Read the model definition and answer for the solid it produces. Units are mm, in the model's axes. Coordinates: 2 decimals unless noted, no trailing zeros. Write each loop counter-clockwise with the first axis right and the second up, starting at its lowest first coordinate (ties: lowest second). Pieces come first, ordered by that corner, then holes.
(1) The part is cut by section B-B, the plane z = 29.5. State how many separate pieces and enclosed holes the cut face has, and give its area (3 significant figures).
(2) The part is cut by section C-C, the plane x = 0. Determine the outline of the cut face in (y, z).
(3) Straight lines are drawn through the part: line 1 along Y through (x, z) = (34, 27.75); line 2 along Y through (x, z) = (-16, 29.25); line 3 along X through (y, z) = (-34, 20). For each, find the intervals that lie inside material, in ascending order.
(4) Given pin 1 (7 mm diameter, centred on x = 34, y = 16, fed in from -Z); pin 2 (2.5 mm diameter, centred on x = 34, y = 16, fed in from +Z); pin 3 (1.5 mm diameter, centred on x = -41.5, z = 22, fed in from +Y); pin 4 (5 mm diameter, centred on y = -11.5, z = 22, fed in from +X), each flat-ended and moving along its own axis, determine where each tip first touches the part or whether it passes through.
(5) The part is cut by section A-A, the plane y = 0. Determine the outline of the cut face in (x, z), and give its area (3 significant figures).
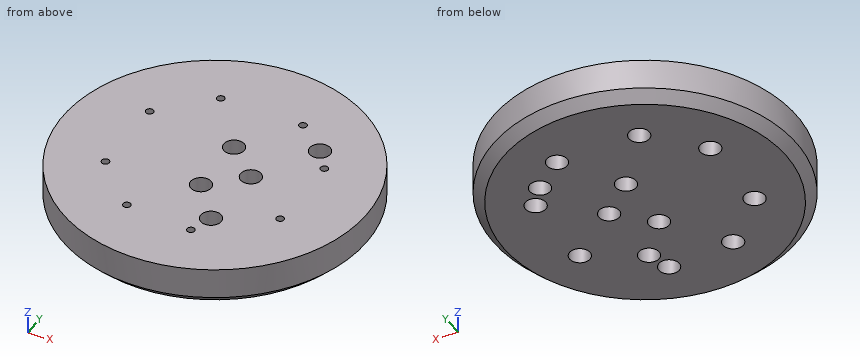
```python
from build123d import *

# Parameters (mm, degrees)
CYLINDER1648_R     = 4
CYLINDER1648_DEPTH = 100
CYLINDER1647_R     = 4
CYLINDER1647_DEPTH = 100
CYLINDER1631_R     = 1.5
CYLINDER1631_DEPTH = 100
CYLINDER1632_R     = 1.5
CYLINDER1632_DEPTH = 100
CYLINDER1633_R     = 1.5
CYLINDER1633_DEPTH = 100
CYLINDER1634_R     = 1.5
CYLINDER1634_DEPTH = 100
CYLINDER1635_R     = 1.5
CYLINDER1635_DEPTH = 100
CYLINDER1636_R     = 1.5
CYLINDER1636_DEPTH = 100
CYLINDER1637_R     = 1.5
CYLINDER1637_DEPTH = 100
CYLINDER1630_R     = 1.5
CYLINDER1630_DEPTH = 100
CYLINDER1651_R     = 4
CYLINDER1651_DEPTH = 100
CYLINDER1649_R     = 4
CYLINDER1649_DEPTH = 100
CYLINDER1652_R     = 4
CYLINDER1652_DEPTH = 100
CYLINDER1653_R     = 4
CYLINDER1653_DEPTH = 100
CYLINDER1654_R     = 4
CYLINDER1654_DEPTH = 100
CYLINDER1655_R     = 4
CYLINDER1655_DEPTH = 100
CYLINDER1656_R     = 4
CYLINDER1656_DEPTH = 100
CYLINDER1650_R     = 4
CYLINDER1650_DEPTH = 100
CYLINDER1640_R     = 4
CYLINDER1640_DEPTH = 20
CYLINDER1641_R     = 4
CYLINDER1641_DEPTH = 20
CYLINDER1642_R     = 4
CYLINDER1642_DEPTH = 20
CYLINDER1643_R     = 4
CYLINDER1643_DEPTH = 40
CYLINDER1644_R     = 4
CYLINDER1644_DEPTH = 40
CYLINDER1645_R     = 4
CYLINDER1645_DEPTH = 40
CYLINDER1646_R     = 4
CYLINDER1646_DEPTH = 40
CYLINDER1639_R     = 4
CYLINDER1639_DEPTH = 20
CYLINDER1638_R     = 59
CYLINDER1638_DEPTH = 16
CHAMFER054_SIZE    = 4


with BuildPart() as obj1:
    # Cylinder1648 → Cylinder1648 (new body)
    with BuildSketch(Plane(origin=(14, 0, -18), x_dir=(1, 0, 0), z_dir=(0, 0, 1))):
        Circle(CYLINDER1648_R)
    extrude(amount=CYLINDER1648_DEPTH)


with BuildPart() as obj2:
    # Cylinder1647 → Cylinder1647 (new body)
    with BuildSketch(Plane(origin=(90, 0, -18), x_dir=(1, 0, 0), z_dir=(0, 0, 1))):
        Circle(CYLINDER1647_R)
    extrude(amount=CYLINDER1647_DEPTH)

    # Compound931: union obj1
    add(obj1.part)


with BuildPart() as obj3:
    # Cylinder1631 → Cylinder1631 (new body)
    with BuildSketch(Plane(origin=(-34, -16, -60), x_dir=(1, 0, 0), z_dir=(0, 0, 1))):
        Circle(CYLINDER1631_R)
    extrude(amount=CYLINDER1631_DEPTH)


with BuildPart() as obj4:
    # Cylinder1632 → Cylinder1632 (new body)
    with BuildSketch(Plane(origin=(34, -16, -60), x_dir=(1, 0, 0), z_dir=(0, 0, 1))):
        Circle(CYLINDER1632_R)
    extrude(amount=CYLINDER1632_DEPTH)


with BuildPart() as obj5:
    # Cylinder1633 → Cylinder1633 (new body)
    with BuildSketch(Plane(origin=(34, 16, -60), x_dir=(1, 0, 0), z_dir=(0, 0, 1))):
        Circle(CYLINDER1633_R)
    extrude(amount=CYLINDER1633_DEPTH)


with BuildPart() as obj6:
    # Cylinder1634 → Cylinder1634 (new body)
    with BuildSketch(Plane(origin=(16, 34, -60), x_dir=(1, 0, 0), z_dir=(0, 0, 1))):
        Circle(CYLINDER1634_R)
    extrude(amount=CYLINDER1634_DEPTH)


with BuildPart() as obj7:
    # Cylinder1635 → Cylinder1635 (new body)
    with BuildSketch(Plane(origin=(10, -36, -60), x_dir=(1, 0, 0), z_dir=(0, 0, 1))):
        Circle(CYLINDER1635_R)
    extrude(amount=CYLINDER1635_DEPTH)


with BuildPart() as obj8:
    # Cylinder1636 → Cylinder1636 (new body)
    with BuildSketch(Plane(origin=(-16, -34, -60), x_dir=(1, 0, 0), z_dir=(0, 0, 1))):
        Circle(CYLINDER1636_R)
    extrude(amount=CYLINDER1636_DEPTH)


with BuildPart() as obj9:
    # Cylinder1637 → Cylinder1637 (new body)
    with BuildSketch(Plane(origin=(-16, 34, -60), x_dir=(1, 0, 0), z_dir=(0, 0, 1))):
        Circle(CYLINDER1637_R)
    extrude(amount=CYLINDER1637_DEPTH)


with BuildPart() as obj10:
    # Cylinder1630 → Cylinder1630 (new body)
    with BuildSketch(Plane(origin=(-34, 16, -60), x_dir=(1, 0, 0), z_dir=(0, 0, 1))):
        Circle(CYLINDER1630_R)
    extrude(amount=CYLINDER1630_DEPTH)

    # Compound928: union obj3, obj4, obj5, obj6, obj7, obj8, obj9
    add(obj3.part)
    add(obj4.part)
    add(obj5.part)
    add(obj6.part)
    add(obj7.part)
    add(obj8.part)
    add(obj9.part)


with BuildPart() as obj11:
    # Cylinder1651 → Cylinder1651 (new body)
    with BuildSketch(Plane(origin=(-16, 34, -90), x_dir=(1, 0, 0), z_dir=(0, 0, 1))):
        Circle(CYLINDER1651_R)
    extrude(amount=CYLINDER1651_DEPTH)


with BuildPart() as obj12:
    # Cylinder1649 → Cylinder1649 (new body)
    with BuildSketch(Plane(origin=(-16, -34, -90), x_dir=(1, 0, 0), z_dir=(0, 0, 1))):
        Circle(CYLINDER1649_R)
    extrude(amount=CYLINDER1649_DEPTH)


with BuildPart() as obj13:
    # Cylinder1652 → Cylinder1652 (new body)
    with BuildSketch(Plane(origin=(34, -16, -90), x_dir=(1, 0, 0), z_dir=(0, 0, 1))):
        Circle(CYLINDER1652_R)
    extrude(amount=CYLINDER1652_DEPTH)


with BuildPart() as obj14:
    # Cylinder1653 → Cylinder1653 (new body)
    with BuildSketch(Plane(origin=(16, 34, -90), x_dir=(1, 0, 0), z_dir=(0, 0, 1))):
        Circle(CYLINDER1653_R)
    extrude(amount=CYLINDER1653_DEPTH)


with BuildPart() as obj15:
    # Cylinder1654 → Cylinder1654 (new body)
    with BuildSketch(Plane(origin=(10, -36, -90), x_dir=(1, 0, 0), z_dir=(0, 0, 1))):
        Circle(CYLINDER1654_R)
    extrude(amount=CYLINDER1654_DEPTH)


with BuildPart() as obj16:
    # Cylinder1655 → Cylinder1655 (new body)
    with BuildSketch(Plane(origin=(-34, 16, -90), x_dir=(1, 0, 0), z_dir=(0, 0, 1))):
        Circle(CYLINDER1655_R)
    extrude(amount=CYLINDER1655_DEPTH)


with BuildPart() as obj17:
    # Cylinder1656 → Cylinder1656 (new body)
    with BuildSketch(Plane(origin=(34, 16, -90), x_dir=(1, 0, 0), z_dir=(0, 0, 1))):
        Circle(CYLINDER1656_R)
    extrude(amount=CYLINDER1656_DEPTH)


with BuildPart() as obj18:
    # Cylinder1650 → Cylinder1650 (new body)
    with BuildSketch(Plane(origin=(-34, -16, -90), x_dir=(1, 0, 0), z_dir=(0, 0, 1))):
        Circle(CYLINDER1650_R)
    extrude(amount=CYLINDER1650_DEPTH)

    # Compound930: union obj11, obj12, obj13, obj14, obj15, obj16, obj17
    add(obj11.part)
    add(obj12.part)
    add(obj13.part)
    add(obj14.part)
    add(obj15.part)
    add(obj16.part)
    add(obj17.part)


with BuildPart() as obj19:
    # Cylinder1640 → Cylinder1640 (new body)
    with BuildSketch(Plane(origin=(103, 12, -20), x_dir=(1, 0, 0), z_dir=(0, 0, 1))):
        Circle(CYLINDER1640_R)
    extrude(amount=CYLINDER1640_DEPTH)


with BuildPart() as obj20:
    # Cylinder1641 → Cylinder1641 (new body)
    with BuildSketch(Plane(origin=(76, 24, -18), x_dir=(1, 0, 0), z_dir=(0, 0, 1))):
        Circle(CYLINDER1641_R)
    extrude(amount=CYLINDER1641_DEPTH)


with BuildPart() as obj21:
    # Cylinder1642 → Cylinder1642 (new body)
    with BuildSketch(Plane(origin=(91, -27, -18), x_dir=(1, 0, 0), z_dir=(0, 0, 1))):
        Circle(CYLINDER1642_R)
    extrude(amount=CYLINDER1642_DEPTH)


with BuildPart() as obj22:
    # Cylinder1643 → Cylinder1643 (new body)
    with BuildSketch(Plane(origin=(13, -27, -18), x_dir=(1, 0, 0), z_dir=(0, 0, 1))):
        Circle(CYLINDER1643_R)
    extrude(amount=CYLINDER1643_DEPTH)


with BuildPart() as obj23:
    # Cylinder1644 → Cylinder1644 (new body)
    with BuildSketch(Plane(origin=(28, 24, -18), x_dir=(1, 0, 0), z_dir=(0, 0, 1))):
        Circle(CYLINDER1644_R)
    extrude(amount=CYLINDER1644_DEPTH)


with BuildPart() as obj24:
    # Cylinder1645 → Cylinder1645 (new body)
    with BuildSketch(Plane(origin=(1, -12, -18), x_dir=(1, 0, 0), z_dir=(0, 0, 1))):
        Circle(CYLINDER1645_R)
    extrude(amount=CYLINDER1645_DEPTH)


with BuildPart() as obj25:
    # Cylinder1646 → Cylinder1646 (new body)
    with BuildSketch(Plane(origin=(1, 12, -18), x_dir=(1, 0, 0), z_dir=(0, 0, 1))):
        Circle(CYLINDER1646_R)
    extrude(amount=CYLINDER1646_DEPTH)


with BuildPart() as obj26:
    # Cylinder1639 → Cylinder1639 (new body)
    with BuildSketch(Plane(origin=(103, -12, -20), x_dir=(1, 0, 0), z_dir=(0, 0, 1))):
        Circle(CYLINDER1639_R)
    extrude(amount=CYLINDER1639_DEPTH)

    # Compound929: union obj19, obj20, obj21, obj22, obj23, obj24, obj25
    add(obj19.part)
    add(obj20.part)
    add(obj21.part)
    add(obj22.part)
    add(obj23.part)
    add(obj24.part)
    add(obj25.part)


with BuildPart() as cut575:
    # Cylinder1638 → Cylinder1638 (new body)
    with BuildSketch(Plane.XY.offset(2)):
        Circle(CYLINDER1638_R)
    extrude(amount=CYLINDER1638_DEPTH)

    # Cut572: cut obj26
    add(obj26.part, mode=Mode.SUBTRACT)

    # Cut573: cut obj18
    add(obj18.part, mode=Mode.SUBTRACT)

    # Cut574: cut obj10
    add(obj10.part, mode=Mode.SUBTRACT)

    # Chamfer054
    chamfer054_edges = [cut575.edges().sort_by_distance(p)[0] for p in [
        (-59, 0, 2),
    ]]
    chamfer(chamfer054_edges, length=CHAMFER054_SIZE)

    # Cut575: cut obj2
    add(obj2.part, mode=Mode.SUBTRACT)


with BuildPart() as cut575_1:
    # Cut575 placement: moved
    add(cut575.part.moved(Location((0, 0, 14))))


solid = cut575_1.part
```
Computed:
1. separate pieces: 1
1. enclosed holes: 13
1. area: 10,600 mm2
2. outline: (-59, 20) - (-55, 16) - (-15.87, 16) - (-15.87, 32) - (-59, 32) - close; (-8.13, 16) - (8.13, 16) - (8.13, 32) - (-8.13, 32) - close; (15.87, 16) - (55, 16) - (59, 20) - (59, 32) - (15.87, 32) - close
3. line 1: y = -48.22 to -17.5, -14.5 to 14.5, 17.5 to 48.22
3. line 2: y = -56.79 to -35.5, -32.5 to 32.5, 35.5 to 56.79
3. line 3: x = -48.22 to -20, -12 to 6.54, 13.46 to 48.22
4. pin 1: stops at z = 24
4. pin 2: passes through
4. pin 3: stops at y = 42.67
4. pin 4: stops at x = 58.31
5. outline: (-59, 20) - (-55, 16) - (10, 16) - (10, 32) - (-59, 32) - close; (18, 16) - (55, 16) - (59, 20) - (59, 32) - (18, 32) - close
5. area: 1,740 mm2
